Read the model definition and answer for the solid it produces. Units are mm, in the model's axes. Face numbers are marked on the shaded views. A direction names the side the tool comes from. Round coordinates to 2 decimals unless told otherwise and drop trailing zeros. Write each loop counter-clockwise with the first axis right and the second up, starting at its lowest first coordinate (ties: lowest second). Pieces come first, ordered by that corner, then holes. Notation, with made-up numbers: (-22, 75) - (-5, 75) arc R13 cw to (-5, 80) - close; hole circle Ø11 at (-36, 78.25). An arc over 180 degrees is marked (long way). Use one line per item in the form item = value. Start each with the question number.
1) The part is cut by section C-C, the plane x = 0. Give the vertices of the cut face in (y, z) (3 decimals), plus the area to 3 significant figures.
2) Consider line 1 along Y through (x, z) = (-45.72, 5) (3 decimals); line 2 along X through (y, z) = (-49, 12); line 3 along Y through (x, z) = (35.5, 5.45) (3 decimals). Determine where each line is inside the solid, lowest interval first. Write a range as from..to.
3) For the marked faces 4, 5, 6 and 7, determine the directions among +Z, -Z, +X, -X, +Y, -Y from which every point of the face is accessible in a straight line to the end or side of a thin tool.
4) Each of these flat-tipped pins is pushed along its axis until it touches: pin 1 (7.5 mm diameter, centred on x = 21.5, z = 5.5, fed in from -Y); pin 2 (3.5 mm diameter, centred on x = -11, z = 2.5, fed in from -Y); pin 3 (2 mm diameter, centred on x = -57.5, z = 11.5, fed in from -Y); pin 4 (3.5 mm diameter, centred on x = 36.8, y = 24.15, fed in from -Z). Where does it stop, or does it pass through?
5) The part is cut by section A-A, the plane y = 0. Give the vertices of the cut face in (x, z) (3 decimals).
6) The part is cut by section B-B, the plane x = 53.3. Give the vertices of the cut face in (y, z) (3 decimals).
7) For a pull along Y with two mould halves and no side action, classify the marked faces 1, 2 and 3 as released by +Y, released by -Y, zero draft, split by the parting line, or undercut.
8) The part is cut by section D-D, the plane y = -36.5. Give the vertices of the cut face in (x, z), plus the area to 3 significant figures.
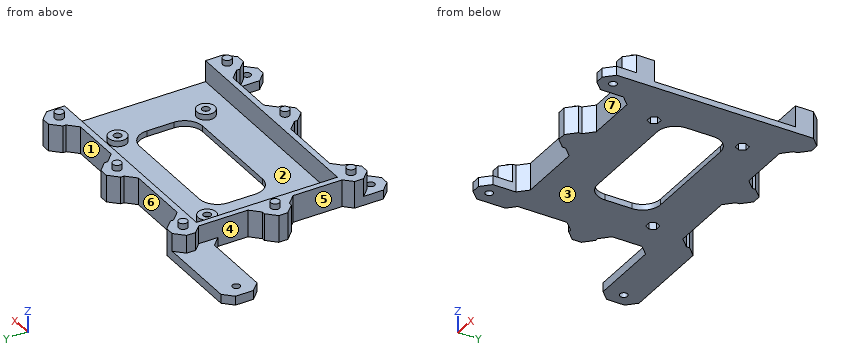
from build123d import *

# Parameters (mm, degrees)
F0_W          = 121.6
F0_H          = 78.3
F0_R          = 2.125
F1_DEPTH      = 3.2
F2_R          = 5
F2_R_2        = 2.125
F3_DEPTH      = 3.2
F5_DEPTH      = 4
F7_DEPTH      = 15
F8_R          = 2.425
F9_DEPTH      = 3.2
F10_T1_DEPTH  = 15
F10_T3_DEPTH  = 40.7168298797
F10_T8_DEPTH  = 40.7168298797
F10_T13_DEPTH = 40.7168298797
F11_W         = 15
F11_H         = 17.8
F11_R         = 2.125
F11_W_2       = 50
F11_H_2       = 20
F12_DEPTH     = 5
F13_SIZE      = 5


# Not quite as in the source:
# - a fillet or chamfer that OpenCascade refuses, or shapes differently, is made with other operations: its cross-section is extruded or revolved along the edge and cut away or added
# - a feature names something its author has since deleted; it is built from what else it names


with BuildPart() as f1:
    # F0 (on Top) → F1 (new body)
    with BuildSketch(Plane.XY):
        Rectangle(F0_W, F0_H)
        with Locations((35.5, -24.05)):
            Circle(F0_R, mode=Mode.SUBTRACT)
        with BuildLine():
            ThreePointArc((37.5, -7.5), (34.5710678119, -14.5710678119), (27.5, -17.5))
            Line((27.5, -17.5), (-27.5, -17.5))
            ThreePointArc((-27.5, -17.5), (-34.5710678119, -14.5710678119), (-37.5, -7.5))
            Line((-37.5, -7.5), (-37.5, 7.5))
            ThreePointArc((-37.5, 7.5), (-34.5710678119, 14.5710678119), (-27.5, 17.5))
            Line((-27.5, 17.5), (27.5, 17.5))
            ThreePointArc((27.5, 17.5), (34.5710678119, 14.5710678119), (37.5, 7.5))
            Line((37.5, 7.5), (37.5, -7.5))
        make_face(mode=Mode.SUBTRACT)
        with Locations((-45.72, 24.15)):
            Circle(F0_R, mode=Mode.SUBTRACT)
        with Locations((36.8, 24.15)):
            Circle(F0_R, mode=Mode.SUBTRACT)
    extrude(amount=F1_DEPTH)

    # F2 (on face) → F3 (join)
    with BuildSketch(Plane.XY.offset(3.2)):
        with Locations((-45.72, 24.15)):
            Circle(F2_R)
        with Locations((-45.72, 24.15)):
            Circle(F2_R_2, mode=Mode.SUBTRACT)
        with Locations((36.8, 24.15)):
            Circle(F2_R)
        with Locations((36.8, 24.15)):
            Circle(F2_R_2, mode=Mode.SUBTRACT)
        with Locations((35.5, -24.05)):
            Circle(F2_R)
        with Locations((35.5, -24.05)):
            Circle(F2_R_2, mode=Mode.SUBTRACT)
    extrude(amount=F3_DEPTH)

    # F4 (on face) → F5 (cut)
    with BuildSketch(Plane(origin=(0, 0, 0), x_dir=(1, 0, 0), z_dir=(0, 0, -1))):
        Polygon((-44.0312504626, -21.225), (-47.4087495374, -21.225), (-49.0974990748, -24.15), (-47.4087495374, -27.075), (-44.0312504626, -27.075), (-42.3425009252, -24.15), align=None)
        Polygon((38.4887495374, -21.225), (35.1112504626, -21.225), (33.4225009252, -24.15), (35.1112504626, -27.075), (38.4887495374, -27.075), (40.1774990748, -24.15), align=None)
        Polygon((33.8112504626, 21.125), (37.1887495374, 21.125), (38.8774990748, 24.05), (37.1887495374, 26.975), (33.8112504626, 26.975), (32.1225009252, 24.05), align=None)
    extrude(amount=-F5_DEPTH, mode=Mode.SUBTRACT)

    # F6 (on Top) → F7 (join)
    with BuildSketch(Plane.XY):
        Polygon((-60.8, 39.15), (60.8, 39.15), (60.8, 54.15), (45.8, 54.15), (45.8, 42.35), (7.5, 42.35), (7.5, 54.15), (-7.5, 54.15), (-7.5, 42.35), (-53.3, 42.35), (-53.3, 54.15), (-68.3, 54.15), (-68.3, 39.15), (-64, 39.15), (-64, 7.5), (-75.8, 7.5), (-75.8, -7.5), (-64, -7.5), (-64, -39.15), (-68.3, -39.15), (-68.3, -54.15), (-53.3, -54.15), (-53.3, -42.35), (-7.5, -42.35), (-7.5, -54.15), (7.5, -54.15), (7.5, -42.35), (45.8, -42.35), (45.8, -54.15), (60.8, -54.15), (60.8, -39.15), (-60.8, -39.15), align=None)
    extrude(amount=F7_DEPTH)

    # F8 (on face) → F9 (join)
    with BuildSketch(Plane.XY.offset(15)):
        with Locations((53.3, 46.65)):
            Circle(F8_R)
        with Locations((0, 46.65)):
            Circle(F8_R)
        with Locations((-60.8, 46.65)):
            Circle(F8_R)
        with Locations((-68.3, 0)):
            Circle(F8_R)
        with Locations((-60.8, -46.65)):
            Circle(F8_R)
        with Locations((0, -46.65)):
            Circle(F8_R)
        with Locations((53.3, -46.65)):
            Circle(F8_R)
    extrude(amount=F9_DEPTH)

    # F10: chamfer of 5 on 26 edges, made by hand

    # F10_s2 → F10_t1 (join)
    with BuildSketch(Plane.XY):
        Polygon((-12.5, -42.35), (-7.5, -47.35), (-7.5, -42.35), align=None)
        Polygon((7.5, -47.35), (12.5, -42.35), (7.5, -42.35), align=None)
        Polygon((40.8, -42.35), (45.8, -47.35), (45.8, -42.35), align=None)
        Polygon((-53.3, -47.35), (-48.3, -42.35), (-53.3, -42.35), align=None)
        Polygon((-69, -7.5), (-64, -12.5), (-64, -7.5), align=None)
        Polygon((-64, 12.5), (-69, 7.5), (-64, 7.5), align=None)
        Polygon((-48.3, 42.35), (-53.3, 47.35), (-53.3, 42.35), align=None)
        Polygon((-7.5, 47.35), (-12.5, 42.35), (-7.5, 42.35), align=None)
        Polygon((45.8, 47.35), (40.8, 42.35), (45.8, 42.35), align=None)
        Polygon((12.5, 42.35), (7.5, 47.35), (7.5, 42.35), align=None)
    extrude(amount=F10_T1_DEPTH)

    # F10_s4 → F10_t3 (cut)
    with BuildSketch(Plane.XY.offset(-12.8584149398)):
        Polygon((-75.8, -2.5), (-70.8, -7.5), (-75.8, -7.5), align=None)
        Polygon((-70.8, 7.5), (-75.8, 2.5), (-75.8, 7.5), align=None)
        Polygon((-63.3, 54.15), (-68.3, 49.15), (-68.3, 54.15), align=None)
        Polygon((-53.3, 49.15), (-58.3, 54.15), (-53.3, 54.15), align=None)
        Polygon((-2.5, 54.15), (-7.5, 49.15), (-7.5, 54.15), align=None)
        Polygon((7.5, 49.15), (2.5, 54.15), (7.5, 54.15), align=None)
        Polygon((50.8, 54.15), (45.8, 49.15), (45.8, 54.15), align=None)
        Polygon((60.8, 49.15), (55.8, 54.15), (60.8, 54.15), align=None)
        Polygon((60.8, -49.15), (55.8, -54.15), (60.8, -54.15), align=None)
        Polygon((50.8, -54.15), (45.8, -49.15), (45.8, -54.15), align=None)
        Polygon((2.5, -54.15), (7.5, -49.15), (7.5, -54.15), align=None)
        Polygon((-7.5, -49.15), (-2.5, -54.15), (-7.5, -54.15), align=None)
        Polygon((-58.3, -54.15), (-53.3, -49.15), (-53.3, -54.15), align=None)
        Polygon((-68.3, -49.15), (-63.3, -54.15), (-68.3, -54.15), align=None)
    extrude(amount=F10_T3_DEPTH, mode=Mode.SUBTRACT)


with BuildPart() as f10_tool6:
    # F10_s7 → F10_t8 (new body)
    with BuildSketch(Plane.XY.offset(-12.8584149398)):
        Polygon((-68.3, 44.15), (-63.3, 39.15), (-68.3, 39.15), align=None)
    extrude(amount=F10_T8_DEPTH)

    split(bisect_by=Plane.YZ.offset(-64), keep=Keep.BOTTOM)


with BuildPart() as f1_1:
    add(f1.part)

    # F10_t5: cut F10_tool6
    add(f10_tool6.part, mode=Mode.SUBTRACT)


with BuildPart() as f10_tool11:
    # F10_s12 → F10_t13 (new body)
    with BuildSketch(Plane.XY.offset(-12.8584149398)):
        Polygon((-63.3, -39.15), (-68.3, -44.15), (-68.3, -39.15), align=None)
    extrude(amount=F10_T13_DEPTH)

    split(bisect_by=Plane.YZ.offset(-64), keep=Keep.BOTTOM)


with BuildPart() as f1_2:
    add(f1_1.part)

    # F10_t10: cut F10_tool11
    add(f10_tool11.part, mode=Mode.SUBTRACT)

    # F11 (on Top) → F12 (join)
    with BuildSketch(Plane.XY):
        with Locations((53.3, -56.25)):
            Rectangle(F11_W, F11_H)
        with Locations((53.3, -57.65)):
            Circle(F11_R, mode=Mode.SUBTRACT)
        with Locations((-60.8, -56.25)):
            Rectangle(F11_W, F11_H)
        with Locations((-60.8, -57.65)):
            Circle(F11_R, mode=Mode.SUBTRACT)
        with Locations((-88.225, 44.15)):
            Rectangle(F11_W_2, F11_H_2)
        with Locations((-105.725, 44.15)):
            Circle(F11_R, mode=Mode.SUBTRACT)
    extrude(amount=F12_DEPTH)

    # F13
    f13_edges = [f1_2.edges().sort_by_distance(p)[0] for p in [
        (-68.3, -65.15, 2.5),
        (-53.3, -65.15, 2.5),
        (45.8, -65.15, 2.5),
        (60.8, -65.15, 2.5),
        (-113.225, 54.15, 2.5),
        (-113.225, 34.15, 2.5),
        (-64, 34.15, 2.5),
    ]]
    chamfer(f13_edges, length=F13_SIZE)


solid = f1_2.part
Geometry results:
q1.outline = (-54.15, 0) - (-17.5, 0) - (-17.5, 3.2) - (-39.15, 3.2) - (-39.15, 15) - (-44.225, 15) - (-44.225, 18.2) - (-49.075, 18.2) - (-49.075, 15) - (-54.15, 15) - close; (17.5, 0) - (54.15, 0) - (54.15, 15) - (49.075, 15) - (49.075, 18.2) - (44.225, 18.2) - (44.225, 15) - (39.15, 15) - (39.15, 3.2) - (17.5, 3.2) - close
q1.area = 620 mm2
q2.line_1 = -42.35..-39.15, 19.15..22.025, 26.275..29.15, 39.15..42.35
q2.line_2 = -68.3..-53.3, -7.5..7.5, 45.8..60.8
q2.line_3 = -42.35..-39.15, -29.05..-26.175, -21.925..-19.05, 19.322..22.469, 25.831..28.978, 39.15..42.35
q3.face_4 = +Z, -X
q3.face_5 = +Z, -Z, -X
q3.face_6 = +Z, -Z, +Y
q3.face_7 = +Z, -Z, -Y
q4.pin_1 = -42.35
q4.pin_2 = -45.6
q4.pin_3 = -54.15
q4.pin_4 = through
q5.outline = (-75.8, 0) - (-37.5, 0) - (-37.5, 3.2) - (-60.8, 3.2) - (-60.8, 15) - (-65.875, 15) - (-65.875, 18.2) - (-70.725, 18.2) - (-70.725, 15) - (-75.8, 15) - close; (37.5, 0) - (60.8, 0) - (60.8, 3.2) - (37.5, 3.2) - close
q6.outline = (-65.15, 0) - (-59.775, 0) - (-59.775, 5) - (-65.15, 5) - close; (-55.525, 0) - (54.15, 0) - (54.15, 15) - (49.075, 15) - (49.075, 18.2) - (44.225, 18.2) - (44.225, 15) - (39.15, 15) - (39.15, 3.2) - (-39.15, 3.2) - (-39.15, 15) - (-44.225, 15) - (-44.225, 18.2) - (-49.075, 18.2) - (-49.075, 15) - (-54.15, 15) - (-54.15, 5) - (-55.525, 5) - close
q7.face_1 = released by +Y
q7.face_2 = undercut
q7.face_3 = zero draft
q8.outline = (-64, 0) - (60.8, 0) - (60.8, 3.2) - (-60.8, 3.2) - (-60.8, 15) - (-64, 15) - close
q8.area = 437 mm2
